Input: dimensioned drawing with shaded views. Units: mm. Origin: part minimum x, y, z. A direction names the side the tool comes from. Round coordinates to 2 decimals unless told otherwise and drop trailing zeros. Order: outer loops, then holes, each group sorted by start corner. A loop starts at its lowest first (then second) coordinate and runs counter-clockwise, first axis right, second up.
Item 1: Cut plane B-B on x = 15. Output: boundary loops of the cut face in (y, z) (3 decimals), then the cut area to 3 significant figures.
Item 2: Cut plane C-C on z = 2.25. Output: boundary loops of the cut face in (x, y) (3 decimals), then the cut area to 3 significant figures.
Item 3: Mould query, pull axis Y, two halves, no side actions, for the marked faces 1, 2, 3 and 4. Classes: released by +Y, released by -Y, zero draft, split by the parting line, or undercut.
Item 4: Line query: L1, parallel to Y at x = 5, z = 1; L2, parallel to Y at x = 8, z = 3 (3 decimals); L3, parallel to Y at x = 11, z = 6.75 (3 decimals). Output: solid intervals per line, ascending.
Item 5: Reachability of the marked faces 5, 6 and 7 from +Z, -Z, +X, -X, +Y, -Y: full face, straight path, thin tool, end or side. Return the list, or none.
Item 6: Cut plane A-A on y = 16.51. Output: boundary loops of the cut face in (x, z) (3 decimals).
Item 7: Cut plane D-D on y = 38.5. Output: boundary loops of the cut face in (x, z) (3 decimals).
Item 8: First-contact query: pin 1 (4 mm diameter, centred on y = 129.5, z = 4, fed in from +X) (3 decimals). Flat tip, straight axial feed; report the tip coordinate or a pass-through.
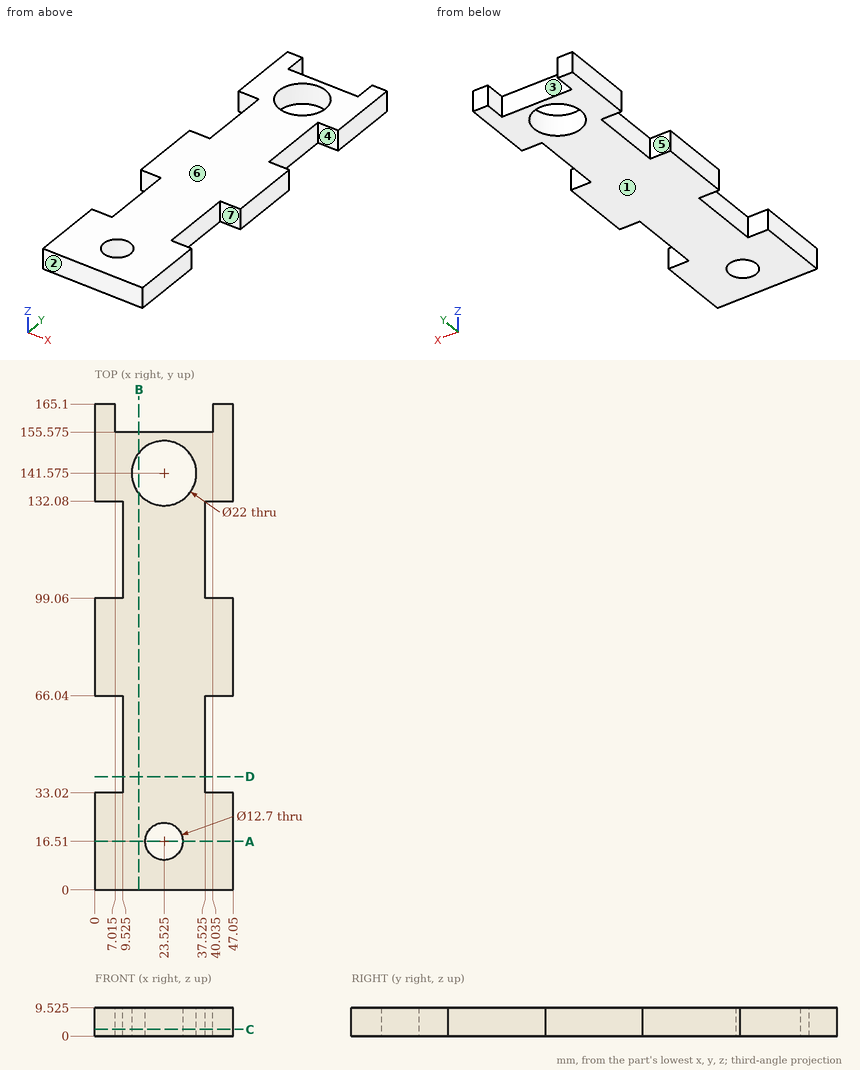
From the geometry:
1. outline: (0, 0) - (134.623, 0) - (134.623, 9.525) - (0, 9.525) - close; (148.527, 0) - (155.575, 0) - (155.575, 9.525) - (148.527, 9.525) - close
1. area: 1,350 mm2
2. outline: (0, 0) - (47.05, 0) - (47.05, 33.02) - (37.525, 33.02) - (37.525, 66.04) - (47.05, 66.04) - (47.05, 99.06) - (37.525, 99.06) - (37.525, 132.08) - (47.05, 132.08) - (47.05, 165.1) - (40.035, 165.1) - (40.035, 155.575) - (7.015, 155.575) - (7.015, 165.1) - (0, 165.1) - (0, 132.08) - (9.525, 132.08) - (9.525, 99.06) - (0, 99.06) - (0, 66.04) - (9.525, 66.04) - (9.525, 33.02) - (0, 33.02) - close; hole circle Ø22 at (23.525, 141.575); hole circle Ø12.7 at (23.525, 16.51)
2. area: 5,690 mm2
3. face 1: zero draft
3. face 2: released by -Y
3. face 3: released by +Y
3. face 4: undercut
4. L1: y = 0 to 33.02, 66.04 to 99.06, 132.08 to 165.1
4. L2: y = 0 to 33.02, 66.04 to 99.06, 132.08 to 155.575
4. L3: y = 0 to 155.575
5. face 5: +Z, -Z, -X
5. face 6: +Z, +X, -X, +Y, -Y
5. face 7: +Z, -Z, +X
6. outline: (0, 0) - (17.175, 0) - (17.175, 9.525) - (0, 9.525) - close; (29.875, 0) - (47.05, 0) - (47.05, 9.525) - (29.875, 9.525) - close
7. outline: (9.525, 0) - (37.525, 0) - (37.525, 9.525) - (9.525, 9.525) - close
8. pin 1: stops at x = 37.525
